For this review, take the finished solid that the model builds, in its own axes (mm). Face numbers are marked on the shaded views. A direction names the side the tool comes from. Give positions to 0.01 mm unless a question says otherwise; leave off trailing zeros. Write each loop counter-clockwise with the first axis right and the second up, starting at its lowest first coordinate (ties: lowest second). Pieces come first, ordered by that corner, then holes.
Q1. Machinability: for the marked faces 4 and 5, which of the approach directions +Z, -Z, +X, -X, +Y, -Y give a long, thin tool a straight path to every point of the face, cutting with its end or side? Answer none if there is none.
Q2. We need section A-A (x = -43.18). Write out the cut boundary in (y, z), then the cut area to 3 significant figures.
Q3. We need section D-D (y = 10.5). Write out the cut boundary in (x, z) (1 decimal).
Q4. Insertion check: P1, Ø1.5, axis at x = -2.5, y = 9.5, coming from the +Z side; P2, Ø2, axis at x = -21.5, y = -6.5, coming from the -Z side; P3, Ø5, axis at x = -16, z = 8, coming from the +Y side. Each pin has a flat end and moves straight along its axis. Give the tip position at first contact, or say it passes through.
Q5. Mouldability with a two-part tool opening along X and no side actions: class the marked faces 1, 2 and 3 as released by +X, released by -X, zero draft, split by the parting line, or undercut.
Q6. We need section C-C (y = -4). Write out the cut boundary in (x, z), then the cut area to 3 significant figures.
Q7. We need section B-B (z = 25.4). Write out the cut boundary in (x, y), then the cut area to 3 significant figures.
Q8. For line 1 (X direction, y = -7.8, z = 0); line 2 (Z direction, x = -17.78, y = -8.25); line 3 (Z direction, x = -17, y = -9), list the stretches that pass through material, from the lowest coordinate up.
```python
from build123d import *

# Parameters (mm, degrees)
SKETCH2_R          = 2.2479
CUT_EXTRUDE1_DEPTH = 4.81
FILLET1_R          = 5.08


with BuildPart() as part:
    # Sketch1 → Revolve1 (revolve)
    with BuildSketch(Plane.XY):
        Polygon((0, 0), (2.54, 20.32), (6.35, 20.32), (3.01625, -6.35), (12.7, -6.35), (12.7, -10.16), (0, -10.16), (0, -5.08), (-17.78, -5.08), (-17.78, 0), align=None)
    revolve(axis=Axis((-17.78, -37.211045685, 0), (0, 1, 0)))

    # Sketch2 → Cut-Extrude1 (cut, through all)
    with BuildSketch(Plane(origin=(0, -6.35, 0), x_dir=(1, 0, 0), z_dir=(0, 1, 0))):
        with Locations((-17.78, -25.4)):
            Circle(SKETCH2_R)
        with Locations((-17.78, 25.4)):
            Circle(SKETCH2_R)
        with Locations((-43.18, 0)):
            Circle(SKETCH2_R)
        with Locations((7.62, 0)):
            Circle(SKETCH2_R)
        with BuildLine():
            Line((12.03120427, -6.35), (2.559936246, -4.332552083))
            ThreePointArc((2.559936246, -4.332552083), (-3.074830602, -14.705169398), (-13.447447917, -20.339936246))
            Line((-13.447447917, -20.339936246), (-11.43, -29.81120427))
            ThreePointArc((-11.43, -29.81120427), (3.772614691, -21.552614691), (12.03120427, -6.35))
        make_face()
        with BuildLine():
            Line((-13.447447917, 20.339936246), (-11.43, 29.81120427))
            ThreePointArc((-11.43, 29.81120427), (3.772614691, 21.552614691), (12.03120427, 6.35))
            Line((12.03120427, 6.35), (2.559936246, 4.332552083))
            ThreePointArc((2.559936246, 4.332552083), (-3.074830602, 14.705169398), (-13.447447917, 20.339936246))
        make_face()
        with BuildLine():
            Line((-22.112552083, -20.339936246), (-24.13, -29.81120427))
            ThreePointArc((-24.13, -29.81120427), (-39.332614691, -21.552614691), (-47.59120427, -6.35))
            Line((-47.59120427, -6.35), (-38.119936246, -4.332552083))
            ThreePointArc((-38.119936246, -4.332552083), (-32.485169398, -14.705169398), (-22.112552083, -20.339936246))
        make_face()
        with BuildLine():
            Line((-47.59120427, 6.35), (-38.119936246, 4.332552083))
            ThreePointArc((-38.119936246, 4.332552083), (-32.485169398, 14.705169398), (-22.112552083, 20.339936246))
            Line((-22.112552083, 20.339936246), (-24.13, 29.81120427))
            ThreePointArc((-24.13, 29.81120427), (-39.332614691, 21.552614691), (-47.59120427, 6.35))
        make_face()
    extrude(amount=-CUT_EXTRUDE1_DEPTH, mode=Mode.SUBTRACT)

    # Fillet1
    fillet1_edges = [part.edges().sort_by_distance(p)[0] for p in [
        (-24.13, -8.255, 29.81120427),
        (-47.59120427, -8.255, 6.35),
        (-11.43, -8.255, -29.81120427),
        (12.03120427, -8.255, -6.35),
        (-47.59120427, -8.255, -6.35),
        (-24.13, -8.255, -29.81120427),
        (12.03120427, -8.255, 6.35),
        (-11.43, -8.255, 29.81120427),
    ]]
    fillet(fillet1_edges, radius=FILLET1_R)


solid = part.part
```
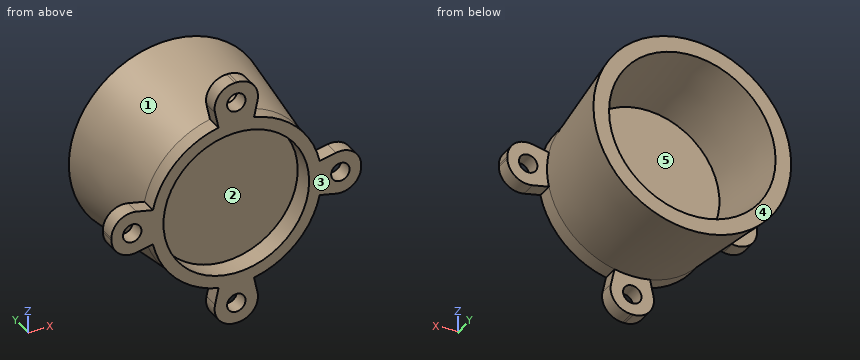
Computed:
1. face 4: +Z, -Z, +X, -X, +Y
1. face 5: +Y
2. outline: (-10.16, -5.3) - (-6.35, -5.3) - (-6.35, -2.25) - (-10.16, -2.25) - close; (-10.16, 2.25) - (-6.35, 2.25) - (-6.35, 5.3) - (-10.16, 5.3) - close
2. area: 23.2 mm2
3. outline: circle Ø45.8 at (-17.8, 0); hole circle Ø38.2 at (-17.8, 0)
4. P1: stops at z = 17.55
4. P2: stops at z = -29.82
4. P3: stops at y = 0
5. face 1: split by the parting line
5. face 2: undercut
5. face 3: zero draft
6. outline: circle Ø42.18 at (-17.78, 0)
6. area: 1,400 mm2
7. outline: (-23.08, -10.16) - (-20.03, -10.16) - (-20.03, -6.35) - (-23.08, -6.35) - close; (-15.53, -10.16) - (-12.48, -10.16) - (-12.48, -6.35) - (-15.53, -6.35) - close
7. area: 23.2 mm2
8. line 1: x = -48.26 to -45.43, -40.93 to -35.56, 0 to 5.37, 9.87 to 12.7
8. line 2: z = -30.48 to -27.65, -23.15 to -17.78, 17.78 to 23.15, 27.65 to 30.48
8. line 3: z = -30.45 to -27.51, -23.29 to -17.76, 17.76 to 23.29, 27.51 to 30.45
